Part model, mm, in its own coordinate system. Round coordinates to 2 decimals unless told otherwise and drop trailing zeros. Write each loop counter-clockwise with the first axis right and the second up, starting at its lowest first coordinate (ties: lowest second). Pieces come first, ordered by that corner, then holes. Notation, with made-up numbers: M 1,-5 L 8,-5 A24 ccw 8,16 Z; hole C 30,22.25 d8. An arc over 180 degrees is marked long. Use a Markdown table: item, result. Add a question column.
1) Drop flat-ended pins along their axis: P1, Ø1, axis at y = 44.5, z = 0.5, coming from the -X side; P2, Ø1, axis at x = 58.5, z = 1, coming from the +Y side; P3, Ø1.5, axis at y = -6.5, z = 2, coming from the -X side; P4, Ø2.5, axis at x = 0, y = -45, coming from the -Z side. Give the stop position or say it passes through.
2) Slice it at C-C on z = 2. Give the number of separate pieces and of enclosed holes in the cut face, plus the area to 3 significant figures.
3) Slice it at B-B on y = 0. Write the cut outline in (x, z).
4) Slice it at D-D on x = 60. Write the cut outline in (y, z).
5) Slice it at A-A on x = -35.5. Write the cut outline in (y, z), plus the area to 3 significant figures.
6) Wall check: probe 1 along X at (y, z) = (-15, 0.4); probe 2 along X at (y, z) = (17, 0.3); probe 3 along X at (y, z) = (-65, 2.2). Give the ranges that are in metal, low to high.
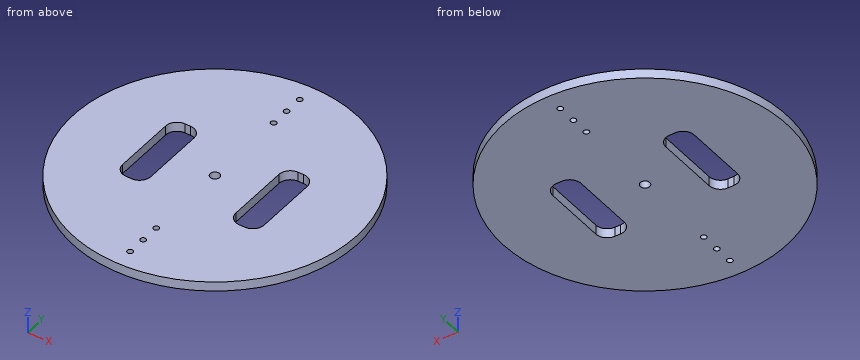
```python
from build123d import *

# Parameters (mm, degrees)
ESBO_O1_R                = 75
RESSALTO_EXTRUS_O1_DEPTH = 5
ESBO_O2_R                = 2.5
CORTE_EXTRUS_O1_DEPTH    = 10
ESBO_O3_R                = 1.5
CORTE_EXTRUS_O2_DEPTH    = 10
CORTE_EXTRUS_O3_DEPTH    = 6


with BuildPart() as part:
    # Esboço1 → Ressalto-extrusão1 (new body)
    with BuildSketch(Plane.XY):
        Circle(ESBO_O1_R)
    extrude(amount=RESSALTO_EXTRUS_O1_DEPTH)

    # Esboço2 → Corte-extrusão1 (cut)
    with BuildSketch(Plane(origin=(0, 0, 0), x_dir=(-1, 0, 0), z_dir=(0, 0, -1))):
        Circle(ESBO_O2_R)
    extrude(amount=-CORTE_EXTRUS_O1_DEPTH, mode=Mode.SUBTRACT)

    # Esboço3 → Corte-extrusão2 (cut)
    with BuildSketch(Plane(origin=(0, 0, 0), x_dir=(-1, 0, 0), z_dir=(0, 0, -1))):
        with Locations((0, -45)):
            Circle(ESBO_O3_R)
        with Locations((0, -55)):
            Circle(ESBO_O3_R)
        with Locations((0, -65)):
            Circle(ESBO_O3_R)
        with Locations((0, 65)):
            Circle(ESBO_O3_R)
        with Locations((0, 55)):
            Circle(ESBO_O3_R)
        with Locations((0, 45)):
            Circle(ESBO_O3_R)
    extrude(amount=-CORTE_EXTRUS_O2_DEPTH, mode=Mode.SUBTRACT)

    # Esboço4 → Corte-extrusão3 (cut, through all)
    with BuildSketch(Plane(origin=(0, 0, 0), x_dir=(-1, 0, 0), z_dir=(0, 0, -1))):
        with BuildLine():
            Line((-31.5, -22.5), (-28.5, -22.5))
            ThreePointArc((-28.5, -22.5), (-24.257359313, -20.742640687), (-22.5, -16.5))
            Line((-22.5, -16.5), (-22.5, 16.5))
            ThreePointArc((-22.5, 16.5), (-24.257359313, 20.742640687), (-28.5, 22.5))
            Line((-28.5, 22.5), (-31.5, 22.5))
            ThreePointArc((-31.5, 22.5), (-35.742640687, 20.742640687), (-37.5, 16.5))
            Line((-37.5, 16.5), (-37.5, -16.5))
            ThreePointArc((-37.5, -16.5), (-35.742640687, -20.742640687), (-31.5, -22.5))
        make_face()
        with BuildLine():
            Line((28.5, -22.5), (31.5, -22.5))
            ThreePointArc((31.5, -22.5), (35.742640687, -20.742640687), (37.5, -16.5))
            Line((37.5, -16.5), (37.5, 16.5))
            ThreePointArc((37.5, 16.5), (35.742640687, 20.742640687), (31.5, 22.5))
            Line((31.5, 22.5), (28.5, 22.5))
            ThreePointArc((28.5, 22.5), (24.257359313, 20.742640687), (22.5, 16.5))
            Line((22.5, 16.5), (22.5, -16.5))
            ThreePointArc((22.5, -16.5), (24.257359313, -20.742640687), (28.5, -22.5))
        make_face()
    extrude(amount=-CORTE_EXTRUS_O3_DEPTH, mode=Mode.SUBTRACT)


solid = part.part
```
Entries:
| question | item | result |
|---|---|---|
| 1 | P1 | stops at x = -60.74 |
| 1 | P2 | stops at y = 47.55 |
| 1 | P3 | stops at x = -74.78 |
| 1 | P4 | passes through |
| 2 | separate pieces | 1 |
| 2 | enclosed holes | 9 |
| 2 | area | 16,300 mm^2 |
| 3 | outline | M -75,0 L -37.5,0 L -37.5,5 L -75,5 Z; M -22.5,0 L -2.5,0 L -2.5,5 L -22.5,5 Z; M 2.5,0 L 22.5,0 L 22.5,5 L 2.5,5 Z; M 37.5,0 L 75,0 L 75,5 L 37.5,5 Z |
| 4 | outline | M -45,0 L 45,0 L 45,5 L -45,5 Z |
| 5 | outline | M -66.07,0 L -20.97,0 L -20.97,5 L -66.07,5 Z; M 20.97,0 L 66.07,0 L 66.07,5 L 20.97,5 Z |
| 5 | area | 451 mm^2 |
| 6 | probe 1 | x = -73.48 to -37.5, -22.5 to 22.5, 37.5 to 73.48 |
| 6 | probe 2 | x = -73.05 to -37.48, -22.52 to 22.52, 37.48 to 73.05 |
| 6 | probe 3 | x = -37.42 to -1.5, 1.5 to 37.42 |
